from build123d import *

# Parameters (mm, degrees)
F0_R     = 50
F1_DEPTH = 50
F2_DEPTH = 10
F4_D     = 60
F5_D     = 40


with BuildPart() as f1:
    # F0 (on Right) → F1 (new body)
    with BuildSketch(Plane.YZ):
        with BuildLine():
            Line((-40, 195.959179), (-200, 0))
            ThreePointArc((-200, 0), (0, -200), (200, 0))
            Line((200, 0), (40, 195.959179))
            ThreePointArc((40, 195.959179), (0, 200), (-40, 195.959179))
        make_face()
        Circle(F0_R, mode=Mode.SUBTRACT)
        Circle(F0_R)
    extrude(amount=-F1_DEPTH)

    # F0 (on Right) → F2 (join)
    with BuildSketch(Plane.YZ):
        Circle(F0_R)
    extrude(amount=F2_DEPTH)

    # F4 (through all)
    with Locations(Plane.YZ.offset(10)):
        with Locations((0, 0)):
            Hole(F4_D / 2)

    # F5 (through all)
    with Locations(Plane.YZ):
        with Locations((0, 130)):
            Hole(F5_D / 2)


solid = f1.part
For this review, take the finished solid that the model builds, in its own axes (mm). A direction names the side the tool comes from. Round coordinates to 2 decimals unless told otherwise and drop trailing zeros. Order: outer loops, then holes, each group sorted by start corner. A loop starts at its lowest first (then second) coordinate and runs counter-clockwise, first axis right, second up. Notation, with made-up numbers: M 88,35 L 99,35 A24 cw 99,50 Z; hole C 55,60 d2. An arc over 180 degrees is marked long. Use a Markdown table: item, result. Add a question column.
Item 1: Mouldability with a two-part tool opening along Z and no side actions: class faces 3 (the flat face through (10, 22, -22)), 4 (the cylindrical face through (-20.42, 29.97, 1.32)), 5 (the cylindrical face through (-24.6, 0.6, 200)), 6 (the cylindrical face through (4.93, 47.69, 15.02)) as released by +Z, released by -Z, zero draft, split by the parting line, or undercut.
Item 2: Tool access review of faces 1 (the cylindrical face through (-25.35, -10.752, 146.864)), 2 (the flat face through (0, 42, -42)): name each direction out of +Z, -Z, +X, -X, +Y, -Y from which nothing blocks a thin tool from reaching the whole face with its end or side.
Item 3: Add section D-D, the plane y = -105. Give the boundary of the cut face in (x, z).
Item 4: Add section A-A, the plane y = 0. Give the boundary of the cut face in (x, z).
Item 5: To check wall thickness, follow line 1 along Z through (x, y) = (-33.5, 0); line 2 along Z through (x, y) = (-40, -2); line 3 along X through (y, z) = (20, -83). State the ranges of each line that lie inside material, in increasing order.
Item 6: Add section C-C, the plane z = 84. Give the boundary of the cut face in (x, y), then the cut area to 3 significant figures.
Item 7: Add section B-B, the plane x = -34.5. Give the boundary of the cut face in (y, z).
Item 8: Insertion check: pin 1 (12 mm diameter, centred on y = 82.5, z = 72.5, fed in from +X); pin 2 (8 mm diameter, centred on x = -3.5, y = 158.5, fed in from -Z); pin 3 (1 mm diameter, centred on x = -34.5, y = 118.5, fed in from -Z); pin 4 (24 mm diameter, centred on y = 0, z = 130, fed in from -X). Each pin has a flat end and moves straight along its axis. Give the tip position at first contact, or say it passes through.
Geometry results:
| question | item | result |
|---|---|---|
| 1 | face 3 | zero draft |
| 1 | face 4 | undercut |
| 1 | face 5 | released by +Z |
| 1 | face 6 | split by the parting line |
| 2 | face 1 | +X, -X |
| 2 | face 2 | +X |
| 3 | outline | M -50,-170.22 L 0,-170.22 L 0,116.35 L -50,116.35 Z |
| 4 | outline | M -50,-200 L 0,-200 L 0,-50 L 10,-50 L 10,-30 L -50,-30 Z; M -50,30 L 10,30 L 10,50 L 0,50 L 0,110 L -50,110 Z; M -50,150 L 0,150 L 0,200 L -50,200 Z |
| 5 | line 1 | z = -200 to -30, 30 to 110, 150 to 200 |
| 5 | line 2 | z = -199.99 to -29.93, 29.93 to 110.1, 149.9 to 199.99 |
| 5 | line 3 | x = -50 to 0 |
| 6 | outline | M -50,-131.41 L 0,-131.41 L 0,131.41 L -50,131.41 Z |
| 6 | area | 13,100 mm² |
| 7 | outline | M -200,0 A200 ccw 200,0 L 40,195.96 A200 ccw -40,195.96 Z; hole C 0,0 d60; hole C 0,130 d40 |
| 8 | pin 1 | stops at x = 0 |
| 8 | pin 2 | stops at z = -127 |
| 8 | pin 3 | stops at z = -161.48 |
| 8 | pin 4 | passes through |
